```python
from build123d import *

# Parameters (mm, degrees)
SKETCH1_W                    = 200
SKETCH1_H                    = 110
BASE_FLANGE1_DEPTH           = 1
EDGE_FLANGE1_STRIP_W         = 5.4732
EDGE_FLANGE1_STRIP_H         = 1
EDGE_FLANGE1_STRIP_CUT_DEPTH = 110
EDGE_FLANGE1_DEPTH           = 110
EDGE_FLANGE2_STRIP_W         = 5.4732
EDGE_FLANGE2_STRIP_H         = 1
EDGE_FLANGE2_STRIP_CUT_DEPTH = 110
EDGE_FLANGE2_DEPTH           = 110
CUT_EXTRUDE1_DEPTH           = 207.869524097
CUT_EXTRUDE1_DEPTH_BACK      = 10
SKETCH14_R                   = 1.25
EDGE_FLANGE3_DEPTH           = 196.5268
EDGE_FLANGE3_BEND_DEPTH      = 196.5268
FILLET1_R                    = 5
SKETCH20_R                   = 2.5
CUT_EXTRUDE2_DEPTH           = 116.952576513


# Sheet-metal steps are written as plain solids
with BuildPart() as part:
    # Sketch1 → Base-Flange1 (new body)
    with BuildSketch(Plane.XY):
        Rectangle(SKETCH1_W, SKETCH1_H)
    extrude(amount=-BASE_FLANGE1_DEPTH)

    # Edge-Flange1 strip (across the edge) → Edge-Flange1 strip cut (cut)
    with BuildSketch(Plane(origin=(-100, 55, 0), x_dir=(1, 0, 0), z_dir=(0, -1, 0))):
        with Locations((-1, -0.5)):
            Rectangle(EDGE_FLANGE1_STRIP_W, EDGE_FLANGE1_STRIP_H)
    extrude(amount=EDGE_FLANGE1_STRIP_CUT_DEPTH, mode=Mode.SUBTRACT)

    # Edge-Flange1 section (across the edge) → Edge-Flange1 (add)
    with BuildSketch(Plane(origin=(-100, 55, 0), x_dir=(1, 0, 0), z_dir=(0, -1, 0))):
        with BuildLine():
            Line((0, 0.7366), (0, 13))
            Line((0, 13), (1, 13))
            Line((1, 13), (1, 0.7366))
            ThreePointArc((1, 0.7366), (1.215745145, 0.215745145), (1.7366, 0))
            Line((1.7366, 0), (1.7366, -1))
            ThreePointArc((1.7366, -1), (0.508638364, -0.491361636), (0, 0.7366))
        make_face()
    extrude(amount=EDGE_FLANGE1_DEPTH)

    # Edge-Flange2 strip (across the edge) → Edge-Flange2 strip cut (cut)
    with BuildSketch(Plane(origin=(100, -55, 0), x_dir=(-1, 0, 0), z_dir=(0, 1, 0))):
        with Locations((-1, -0.5)):
            Rectangle(EDGE_FLANGE2_STRIP_W, EDGE_FLANGE2_STRIP_H)
    extrude(amount=EDGE_FLANGE2_STRIP_CUT_DEPTH, mode=Mode.SUBTRACT)

    # Edge-Flange2 section (across the edge) → Edge-Flange2 (add)
    with BuildSketch(Plane(origin=(100, -55, 0), x_dir=(-1, 0, 0), z_dir=(0, 1, 0))):
        with BuildLine():
            Line((0, 0.7366), (0, 13))
            Line((0, 13), (1, 13))
            Line((1, 13), (1, 0.7366))
            ThreePointArc((1, 0.7366), (1.215745145, 0.215745145), (1.7366, 0))
            Line((1.7366, 0), (1.7366, -1))
            ThreePointArc((1.7366, -1), (0.508638364, -0.491361636), (0, 0.7366))
        make_face()
    extrude(amount=EDGE_FLANGE2_DEPTH)

    # Sketch14 → Cut-Extrude1 (cut, two sides: drawn at the far end of the back side and taken through both)
    with BuildSketch(Plane(origin=(-99, 0, 0), x_dir=(0, 0, -1), z_dir=(1, 0, 0)).offset(-CUT_EXTRUDE1_DEPTH_BACK)):
        with Locations(Location((-7.5, -35, 0), (0, 0, 180))):
            Circle(SKETCH14_R)
        with Locations(Location((-7.5, 35, 0), (0, 0, 180))):
            Circle(SKETCH14_R)
    extrude(amount=CUT_EXTRUDE1_DEPTH + CUT_EXTRUDE1_DEPTH_BACK, mode=Mode.SUBTRACT)

    # Edge-Flange3 section (across the edge) → Edge-Flange3 (add)
    with BuildSketch(Plane(origin=(98.2634, -56, -1), x_dir=(0, 1, 0), z_dir=(-1, 0, 0))):
        with BuildLine():
            Line((-1, 1), (-1, 9))
            Line((-1, 9), (0, 9))
            Line((0, 9), (0, 1))
            ThreePointArc((0, 1), (0.292893219, 0.292893219), (1, 0))
            Line((1, 0), (1, -1))
            ThreePointArc((1, -1), (-0.414213562, -0.414213562), (-1, 1))
        make_face()
    extrude(amount=EDGE_FLANGE3_DEPTH)

    # Edge-Flange3 section 2 (across the edge) → Edge-Flange3 bend (add)
    with BuildSketch(Plane(origin=(-98.2634, 56, -1), x_dir=(0, -1, 0), z_dir=(1, 0, 0))):
        with BuildLine():
            Line((-1, 1), (-1, 9))
            Line((-1, 9), (0, 9))
            Line((0, 9), (0, 1))
            ThreePointArc((0, 1), (0.292893219, 0.292893219), (1, 0))
            Line((1, 0), (1, -1))
            ThreePointArc((1, -1), (-0.414213562, -0.414213562), (-1, 1))
        make_face()
    extrude(amount=EDGE_FLANGE3_BEND_DEPTH)

    # Fillet1
    fillet1_edges = [part.edges().sort_by_distance(p)[0] for p in [
        (98.2634, -56.5, -10),
        (-98.2634, -56.5, -10),
        (-98.2634, 56.5, -10),
        (98.2634, 56.5, -10),
        (-99.5, 55, 13),
        (-99.5, -55, 13),
        (99.5, -55, 13),
        (99.5, 55, 13),
    ]]
    fillet(fillet1_edges, radius=FILLET1_R)

    # Sketch20 → Cut-Extrude2 (cut, through all)
    with BuildSketch(Plane(origin=(0, 0, -1), x_dir=(-1, 0, 0), z_dir=(0, 0, -1))):
        with Locations((47.5, 0)):
            Circle(SKETCH20_R)
        with Locations((62.5, 0)):
            Circle(SKETCH20_R)
    extrude(amount=-CUT_EXTRUDE2_DEPTH, mode=Mode.SUBTRACT)


solid = part.part
```
Read the model definition and answer for the solid it produces. Units are mm, in the model's axes. A direction names the side the tool comes from. Coordinates: 2 decimals unless noted, no trailing zeros. Write each loop counter-clockwise with the first axis right and the second up, starting at its lowest first coordinate (ties: lowest second). Pieces come first, ordered by that corner, then holes. Notation, with made-up numbers: (-35.75, 38.25) - (-17.75, 38.25) arc R24 cw to (-17.75, 73.25) - close; hole circle Ø6 at (-7.75, -10). An arc over 180 degrees is marked (long way). Answer as a JSON object with one key per item and string values. Group by question number.
1. A cutting plane is placed at B-B (x = -47.5). Determine the outline of the cut face in (y, z).
2. The mould has two halves that part along X. Classify faces 4 (the flat face through (-100, 1, 7)), 5 (the flat face through (99, -1, 7)), 6 (the flat face through (-1, 57, -6)): +X half, -X half, draft (parallel to the pull), parting line (faces both ways), or undercut.
3. Each of these flat-tipped pins is pushed along its axis until it touches: P1, Ø2, axis at y = -35, z = 7.5, coming from the -X side; P2, Ø0.5, axis at x = -99, z = 3, coming from the -Y side; P3, Ø6, axis at y = -1, z = -2.5, coming from the +X side; P4, Ø1.5, axis at x = -69.5, y = -41.5, coming from the -Z side. Where does it stop, or does it pass through?
4. A cutting plane is placed at A-A (y = 0). Determine the outline of the cut face in (x, z).
5. Consider L1, parallel to Y at x = 99.65, z = 7.5; L2, parallel to X at y = -11, z = 10; L3, parallel to Y at x = -88, z = -4.25. Determine where each line is inside the solid, lowest interval first. Write a range as [from, to].
6. Which of the six approach directions +Z, -Z, +X, -X, +Y, -Y give full straight-line access (tool end or side, diameter ignored) to faces 1 (the cylindrical face through (99.49, 53.57, 11.5)), 2 (the flat face through (-99, 1, 7)), 3 (the flat face through (-1, 56, -6))?
7. A cutting plane is placed at C-C (x = 82). Determine the outline of the cut face in (y, z).
8. A cutting plane is placed at D-D (y = 19). Determine the outline of the cut face in (x, z), plus the area to 3 significant figures.
Worked out:
{
 "1": {"outline": "(-57, -10) - (-56, -10) - (-56, -2) arc R1 cw to (-55, -1) - (-2.5, -1) - (-2.5, 0) - (-55, 0) arc R2 ccw to (-57, -2) - close; (2.5, -1) - (55, -1) arc R1 cw to (56, -2) - (56, -10) - (57, -10) - (57, -2) arc R2 ccw to (55, 0) - (2.5, 0) - close"},
 "2": {"face 4": "-X half", "face 5": "undercut", "face 6": "draft"},
 "3": {"P1": "passes through", "P2": "stops at y = -55", "P3": "stops at x = 99.98", "P4": "stops at z = -1"},
 "4": {"outline": "(-100, 0.74) arc R1.74 ccw to (-98.26, -1) - (-65, -1) - (-65, 0) - (-98.26, 0) arc R0.74 cw to (-99, 0.74) - (-99, 13) - (-100, 13) - close; (-60, -1) - (-50, -1) - (-50, 0) - (-60, 0) - close; (-45, -1) - (98.26, -1) arc R1.74 ccw to (100, 0.74) - (100, 13) - (99, 13) - (99, 0.74) arc R0.74 cw to (98.26, 0) - (-45, 0) - close"},
 "5": {"L1": "y = [-55, -36.25], [-33.75, 33.75], [36.25, 55]", "L2": "x = [-100, -99], [99, 100]", "L3": "y = [-57, -56], [56, 57]"},
 "6": {"face 1": "+Z, +X, -X, +Y", "face 2": "+Z, +Y, -Y", "face 3": "-Z, +X, -X"},
 "7": {"outline": "(-57, -10) - (-56, -10) - (-56, -2) arc R1 cw to (-55, -1) - (55, -1) arc R1 cw to (56, -2) - (56, -10) - (57, -10) - (57, -2) arc R2 ccw to (55, 0) - (-55, 0) arc R2 ccw to (-57, -2) - close"},
 "8": {"outline": "(-100, 0.74) arc R1.74 ccw to (-98.26, -1) - (98.26, -1) arc R1.74 ccw to (100, 0.74) - (100, 13) - (99, 13) - (99, 0.74) arc R0.74 cw to (98.26, 0) - (-98.26, 0) arc R0.74 cw to (-99, 0.74) - (-99, 13) - (-100, 13) - close", "area": "225 mm²"}
}
